For this review, take the finished solid that the model builds, in its own axes (mm). A direction names the side the tool comes from. Round coordinates to 2 decimals unless told otherwise and drop trailing zeros. Order: outer loops, then holes, each group sorted by start corner. A loop starts at its lowest first (then second) coordinate and runs counter-clockwise, first axis right, second up. Notation, with made-up numbers: (-40, -12) -> (-8, -12) arc R21 cw to (-8, -5) -> close; hole circle Ø5 at (-1, 69). An arc over 180 degrees is marked (long way). Answer in a Markdown table with one row per item.
```python
from build123d import *

# Parameters (mm, degrees)
SKETCH_1_W      = 43.2
SKETCH_1_H      = 27.9
EXTRUDE_1_DEPTH = 4.1
SKETCH_2_W      = 8.1
SKETCH_2_H      = 27.9
SKETCH_2_W_2    = 3.9
EXTRUDE_2_DEPTH = 5.4
FILLET_1_R      = 1


with BuildPart() as part:
    # Эскиз1 → Бобышка-Вытянуть1 (new body)
    with BuildSketch(Plane(origin=(0, 0, 0), x_dir=(1, 0, 0), z_dir=(0, 1, 0))):
        Rectangle(SKETCH_1_W, SKETCH_1_H)
    extrude(amount=EXTRUDE_1_DEPTH)

    # Эскиз2 → Бобышка-Вытянуть2 (add)
    with BuildSketch(Plane(origin=(0, 4.1, 0), x_dir=(1, 0, 0), z_dir=(0, 1, 0))):
        Rectangle(SKETCH_2_W, SKETCH_2_H)
        with Locations((-19.65, 0)):
            Rectangle(SKETCH_2_W_2, SKETCH_2_H)
        with Locations((19.65, 0)):
            Rectangle(SKETCH_2_W_2, SKETCH_2_H)
    extrude(amount=EXTRUDE_2_DEPTH)

    # Скругление1
    fillet_1_edges = [part.edges().sort_by_distance(p)[0] for p in [
        (-10.875, 4.1, -13.95),
        (10.875, 4.1, 13.95),
        (4.05, 6.8, 13.95),
        (4.05, 6.8, -13.95),
        (-4.05, 6.8, -13.95),
        (-4.05, 6.8, 13.95),
        (-10.875, 4.1, 13.95),
        (-17.7, 6.8, 13.95),
        (-17.7, 6.8, -13.95),
        (10.875, 4.1, -13.95),
        (17.7, 6.8, -13.95),
        (17.7, 6.8, 13.95),
        (21.6, 4.75, 13.95),
        (-21.6, 4.75, 13.95),
        (-21.6, 4.75, -13.95),
        (21.6, 4.75, -13.95),
    ]]
    fillet(fillet_1_edges, radius=FILLET_1_R)


solid = part.part
```
Q1. Take a section at C-C, the plane x = -10. Write out the cut boundary in (y, z), then the cut area to 3 significant figures.
Answer key:
| item | result |
|---|---|
| outline | (0, -13.95) -> (3.1, -13.95) arc R1 ccw to (4.1, -12.95) -> (4.1, 12.95) arc R1 ccw to (3.1, 13.95) -> (0, 13.95) -> close |
| area | 114 mm^2 |
Q2. Take a section at B-B, the plane z = -6.5. Write out the cut boundary in (x, y).
Answer key:
| item | result |
|---|---|
| outline | (-21.6, 0) -> (21.6, 0) -> (21.6, 9.5) -> (17.7, 9.5) -> (17.7, 4.1) -> (4.05, 4.1) -> (4.05, 9.5) -> (-4.05, 9.5) -> (-4.05, 4.1) -> (-17.7, 4.1) -> (-17.7, 9.5) -> (-21.6, 9.5) -> close |
Q3. The part is to be moulded in two halves that separate along X. For faces 6 (the face through (-21.315, 4.684, -13.649)), 7 (the face through (10.985, 3.815, -13.649)), 8 (the face through (20, 9.5, 0)), say which applies: +X half, -X half, draft (parallel to the pull), parting line (faces both ways), or undercut.
Answer key:
| item | result |
|---|---|
| face 6 | -X half |
| face 7 | undercut |
| face 8 | draft |
Q4. Tool access review of faces 1 (the face through (-20, 9.5, 0)), 2 (the face through (-3.765, 6.345, -13.649)), 3 (the face through (-3.749, 6.345, 13.665)), 4 (the face through (21.315, 4.684, -13.649)), 5 (the face through (4.05, 7, 0)): name each direction out of +Z, -Z, +X, -X, +Y, -Y from which nothing blocks a thin tool from reaching the whole face with its end or side.
Answer key:
| item | result |
|---|---|
| face 1 | +Z, -Z, +X, -X, +Y |
| face 2 | -Z, +Y |
| face 3 | +Z, +Y |
| face 4 | -Z, +X, +Y, -Y |
| face 5 | +Z, -Z, +Y |
Q5. Take a section at A-A, the plane y = 7.5. Write out the cut boundary in (x, z), then the cut area to 3 significant figures.
Answer key:
| item | result |
|---|---|
| outline | (-21.6, -12.95) arc R1 ccw to (-20.6, -13.95) -> (-18.7, -13.95) arc R1 ccw to (-17.7, -12.95) -> (-17.7, 12.95) arc R1 ccw to (-18.7, 13.95) -> (-20.6, 13.95) arc R1 ccw to (-21.6, 12.95) -> close; (-4.05, -12.95) arc R1 ccw to (-3.05, -13.95) -> (3.05, -13.95) arc R1 ccw to (4.05, -12.95) -> (4.05, 12.95) arc R1 ccw to (3.05, 13.95) -> (-3.05, 13.95) arc R1 ccw to (-4.05, 12.95) -> close; (17.7, -12.95) arc R1 ccw to (18.7, -13.95) -> (20.6, -13.95) arc R1 ccw to (21.6, -12.95) -> (21.6, 12.95) arc R1 ccw to (20.6, 13.95) -> (18.7, 13.95) arc R1 ccw to (17.7, 12.95) -> close |
| area | 441 mm^2 |
Q6. To check wall thickness, follow probe 1 along X at (y, z) = (8.25, 9.25); probe 2 along Y at (x, z) = (-11.5, 1.5); probe 3 along Z at (x, y) = (-13, 3.5). State the ranges of each line that lie inside material, in increasing order.
Answer key:
| item | result |
|---|---|
| probe 1 | x = -21.6 to -17.7, -4.05 to 4.05, 17.7 to 21.6 |
| probe 2 | y = 0 to 4.1 |
| probe 3 | z = -13.87 to 13.87 |
Q7. Clearance check with a flat-ended pin moving along its axis: pin 1 Ø2 at (x, y) = (-7.5, 4.5) entering from +Z. State where the tip first meets the part, or that it passes through.
Answer key:
| item | result |
|---|---|
| pin 1 | stops at z = 13.87 |
